from build123d import *

# Parameters (mm, degrees)
CROQUIS1_W                       = 250
CROQUIS1_H                       = 150
SALIENTE_EXTRUIR1_DEPTH          = 110
REDONDEO1_R                      = 15
VACIADO2_T                       = -3
CROQUIS3_W                       = 250
CROQUIS3_H                       = 150
SALIENTE_EXTRUIR2_DEPTH          = 5
REDONDEO2_R                      = 15
CROQUIS4_W                       = 250
CROQUIS4_H                       = 150
CORTAR_EXTRUIR1_DEPTH            = 3
SALIENTE_EXTRUIR3_DEPTH          = 107
REDONDEO3_R                      = 15
TALADRO_DE_MARGEN_PARA_M41_D     = 4.5
TALADRO_DE_MARGEN_PARA_M41_DEPTH = 40
TALADRO_DE_MARGEN_PARA_M41_TIP   = 1.351936393


with BuildPart() as part:
    # Croquis1 → Saliente-Extruir1 (new body)
    with BuildSketch(Plane(origin=(0, 0, 0), x_dir=(1, 0, 0), z_dir=(0, 1, 0))):
        Rectangle(CROQUIS1_W, CROQUIS1_H)
    extrude(amount=SALIENTE_EXTRUIR1_DEPTH)

    # Redondeo1
    redondeo1_edges = [part.edges().sort_by_distance(p)[0] for p in [
        (125, 55, 75),
        (-125, 55, 75),
        (-125, 55, -75),
        (125, 55, -75),
    ]]
    fillet(redondeo1_edges, radius=REDONDEO1_R)

    # Vaciado2
    vaciado2_openings = [part.faces().sort_by_distance(p)[0] for p in [
        (0, 0, 0),
    ]]
    offset(amount=VACIADO2_T, openings=vaciado2_openings, kind=Kind.INTERSECTION)

    # Croquis3 → Saliente-Extruir2 (add)
    with BuildSketch(Plane.XZ):
        Rectangle(CROQUIS3_W, CROQUIS3_H)
    extrude(amount=-SALIENTE_EXTRUIR2_DEPTH)

    # Redondeo2
    redondeo2_edges = [part.edges().sort_by_distance(p)[0] for p in [
        (125, 2.5, 75),
        (125, 2.5, -75),
        (-125, 2.5, -75),
        (-125, 2.5, 75),
    ]]
    fillet(redondeo2_edges, radius=REDONDEO2_R - 0.0001)  # a hair under: the kernel refuses the full size

    # Croquis4 → Cortar-Extruir1 (cut)
    with BuildSketch(Plane(origin=(0, 110, 0), x_dir=(1, 0, 0), z_dir=(0, 1, 0))):
        Rectangle(CROQUIS4_W, CROQUIS4_H)
    extrude(amount=-CORTAR_EXTRUIR1_DEPTH, mode=Mode.SUBTRACT)

    # Croquis5 → Saliente-Extruir3 (add)
    with BuildSketch(Plane(origin=(0, 107, 0), x_dir=(1, 0, 0), z_dir=(0, 1, 0))):
        Polygon((-125, -47), (-125, -75), (-97, -75), align=None)
        Polygon((-97, 75), (-125, 75), (-125, 47), (-122, 50), (-100, 72), align=None)
        Polygon((97, -75), (125, -75), (125, -47), align=None)
        Polygon((97, 75), (125, 47), (125, 75), align=None)
    extrude(amount=-SALIENTE_EXTRUIR3_DEPTH)

    # Redondeo3
    redondeo3_edges = [part.edges().sort_by_distance(p)[0] for p in [
        (-125, 53.5, -75),
        (125, 53.5, 75),
        (-125, 53.5, 75),
        (125, 53.5, -75),
    ]]
    fillet(redondeo3_edges, radius=REDONDEO3_R)

    # Taladro de margen para M41
    with Locations(Plane(origin=(0, 107, 0), x_dir=(1, 0, 0), z_dir=(0, 1, 0))):
        with Locations((-115, 65), (115, 65), (115, -65), (-115, -65)):
            Hole(TALADRO_DE_MARGEN_PARA_M41_D / 2, depth=TALADRO_DE_MARGEN_PARA_M41_DEPTH)
            with Locations((0, 0, -(TALADRO_DE_MARGEN_PARA_M41_DEPTH + TALADRO_DE_MARGEN_PARA_M41_TIP / 2))):  # 118° drill point
                Cone(0, TALADRO_DE_MARGEN_PARA_M41_D / 2, TALADRO_DE_MARGEN_PARA_M41_TIP, mode=Mode.SUBTRACT)


solid = part.part
Geometry: final body of the model. Coordinates: model frame, mm. A direction names the side the tool comes from. Round coordinates to 2 decimals unless told otherwise and drop trailing zeros. Write each loop counter-clockwise with the first axis right and the second up, starting at its lowest first coordinate (ties: lowest second). Pieces come first, ordered by that corner, then holes. Notation, with made-up numbers: M 38,88.25 L 82,88.25 A32 ccw 82,122.25 Z; hole C -18,3.5 d2. An arc over 180 degrees is marked long. Write item = value, one per line.
Item 1: Pin query (flat end, axial travel): P1, Ø4, axis at x = -115, z = 65, coming from the +Y side; P2, Ø12, axis at x = -35.5, z = 44.5, coming from the +Y side; P3, Ø3.5, axis at x = -115, z = -65, coming from the +Y side. Return the tip coordinate at first contact, or that it passes through.
Findings:
P1 = 66.85
P2 = 5
P3 = 66.7
Item 2: Pull-direction query (X, two-part tool) for faces 3 (the face through (-1, 55, 72)), 4 (the face through (-120.72, 52.75, 70.49)), 5 (the face through (-2, 53, -75)); classes: pulls with the +X half, pulls with the -X half, needs draft (parallel to the pull), parting line crosses it, or undercut.
Findings:
face_3 = undercut
face_4 = pulls with the -X half
face_5 = needs draft
Item 3: Access query for faces 1 (the face through (-2, 0, 1)), 2 (the face through (-111, 57, -61)). Directions: +Z, -Z, +X, -X, +Y, -Y. A direction counts if a zero-diameter tool reaches every point of the face in a straight line with its end or side. Return the directions, or none.
Findings:
face_1 = +Z, -Z, +X, -X, -Y
face_2 = +Y
Item 4: Section query D-D on y = 53. Return loops of the section in (x, z), then the cut area to 3 significant figures.
Findings:
outline = M -125,-60 A15 ccw -110,-75 L 110,-75 A15 ccw 125,-60 L 125,60 A15 ccw 110,75 L -110,75 A15 ccw -125,60 Z; hole M -122,-50 L -100,-72 L 100,-72 L 122,-50 L 122,50 L 100,72 L -100,72 L -122,50 Z
area = 3,140 mm^2
Item 5: Material intervals for line 1 along Z through (x, y) = (24.5, 13.5); line 2 along Z through (x, y) = (115, 82); line 3 along X through (y, z) = (54, -18.5), sorted ascending. Write a range as [from, to].
Findings:
line_1 = [-75, -72], [72, 75]
line_2 = [-74.14, -67.25], [-62.75, -57], [57, 62.75], [67.25, 74.14]
line_3 = [-125, -122], [122, 125]
Item 6: Section query B-B on x = 54. Return loops of the section in (y, z).
Findings:
outline = M 0,-75 L 107,-75 L 107,-72 L 5,-72 L 5,72 L 107,72 L 107,75 L 0,75 Z
Item 7: Section query A-A on y = 80. Return loops of the section in (x, z), then the cut area to 3 significant figures.
Findings:
outline = M -125,-60 A15 ccw -110,-75 L 110,-75 A15 ccw 125,-60 L 125,60 A15 ccw 110,75 L -110,75 A15 ccw -125,60 Z; hole M -122,-50 L -100,-72 L 100,-72 L 122,-50 L 122,50 L 100,72 L -100,72 L -122,50 Z; hole C -115,-65 d4.5; hole C -115,65 d4.5; hole C 115,-65 d4.5; hole C 115,65 d4.5
area = 3,080 mm^2
Item 8: Section query C-C on z = 1.5. Return loops of the section in (x, y), then the cut area to 3 significant figures.
Findings:
outline = M -125,0 L 125,0 L 125,107 L 122,107 L 122,5 L -122,5 L -122,107 L -125,107 Z
area = 1,860 mm^2
